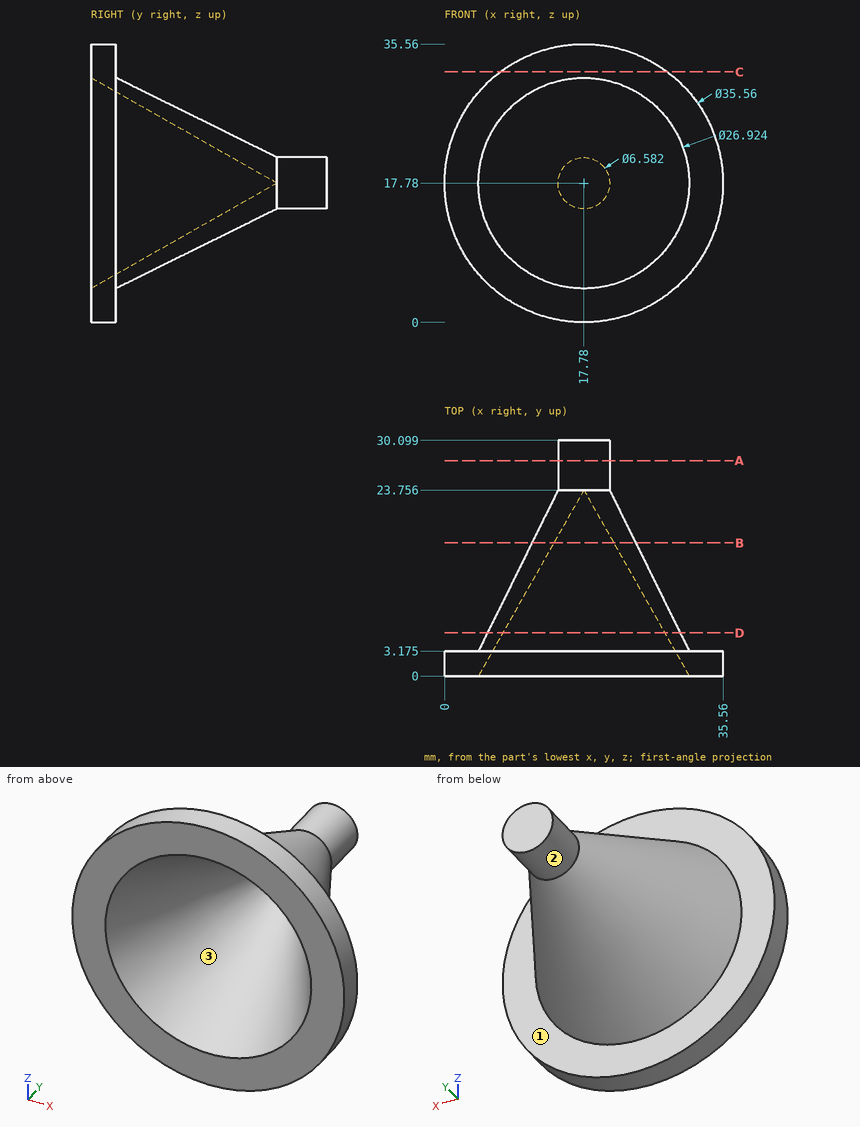
Design review of the part shown in the three views and the two pictorial views. Dimensions are in mm from the part's minimum x, y and z. Give positions to 0.01 mm unless a question says otherwise; leave off trailing zeros. Write each loop counter-clockwise with the first axis right and the second up, starting at its lowest first coordinate (ties: lowest second). Pieces come first, ordered by that corner, then holes.
Item 1: Take a section at D-D (y = 5.5). Give the boundary of the cut face in (x, z) (1 decimal), and give its area (3 significant figures).
Item 2: Take a section at C-C (z = 32). Give the boundary of the cut face in (x, y) (1 decimal).
Item 3: Take a section at A-A (y = 27.5). Give the boundary of the cut face in (x, z).
Item 4: The part is to be moulded in two halves that separate along X. For the marked faces 1, 2 and 3, say which applies: +X half, -X half, draft (parallel to the pull), parting line (faces both ways), or undercut.
Item 5: Insertion check: P1, Ø12, axis at x = 12, y = 23.5, coming from the +Z side; P2, Ø1, axis at x = 11.5, z = 14, coming from the +Y side (1 decimal); P3, Ø3, axis at y = 7.5, z = 25.5, coming from the +X side. Each pin has a flat end and moves straight along its axis. Give the tip position at first contact, or say it passes through.
Item 6: Wall thickness on probe 1 along Z at (x, y) = (18.5, 21.5) (1 decimal); probe 2 along Z at (x, y) = (10, 2) (1 decimal); probe 3 along Y at (x, z) = (23, 33) (1 decimal): over which ranges is each line inside the solid? List them lowest first.
Item 7: Take a section at B-B (y = 17). Give the boundary of the cut face in (x, z).
Established:
1. outline: circle Ø24.6 at (17.8, 17.8); hole circle Ø20.7 at (17.8, 17.8)
1. area: 140 mm2
2. outline: (7.1, 0) - (28.5, 0) - (28.5, 3.2) - (7.1, 3.2) - close
3. outline: circle Ø6.58 at (17.78, 17.78)
4. face 1: draft
4. face 2: parting line
4. face 3: undercut
5. P1: stops at z = 23.14
5. P2: stops at y = 16.6
5. P3: stops at x = 27.58
6. probe 1: z = 13.4 to 16.7, 18.8 to 22.1
6. probe 2: z = 1.8 to 8.2, 27.3 to 33.8
6. probe 3: y = 0 to 3.2
7. outline: circle Ø13.26 at (17.78, 17.78); hole circle Ø7.66 at (17.78, 17.78)
